from build123d import *

# Parameters (mm, degrees)
SKETCH2_W           = 20.32
SKETCH2_H           = 20.32
SKETCH2_R           = 1.325
BOSS_EXTRUDE1_DEPTH = 1.65
SKETCH3_W           = 0.55
SKETCH3_H           = 0.55
LPATTERN1_COUNT     = 4
LPATTERN1_PITCH     = 2.55
LPATTERN1_COL_COUNT = 4
LPATTERN1_COL_PITCH = 2.55
SKETCH5_W           = 17.9
SKETCH5_H           = 2.5
BOSS_EXTRUDE2_DEPTH = 2.75
SKETCH6_W           = 2
SKETCH6_H           = 2.5
SKETCH6_W_2         = 2.5
SKETCH6_H_2         = 3.5
BOSS_EXTRUDE3_DEPTH = 0.5
FILLET1_R           = 2
SKETCH7_W           = 1.7
SKETCH7_H           = 2.7
CUT_EXTRUDE1_DEPTH  = 0.1


with BuildPart() as part:
    # Sketch2 → Boss-Extrude1 (new body)
    with BuildSketch(Plane(origin=(0, 0, 0), x_dir=(1, 0, 0), z_dir=(0, 1, 0))):
        with Locations((10.16, 10.16)):
            Rectangle(SKETCH2_W, SKETCH2_H)
        with Locations((2.54, 17.695)):
            Circle(SKETCH2_R, mode=Mode.SUBTRACT)
        with Locations((17.78, 17.695)):
            Circle(SKETCH2_R, mode=Mode.SUBTRACT)
    extrude(amount=BOSS_EXTRUDE1_DEPTH)

    # Sweep1: sweep along a path in Sketch4
    with BuildLine(Plane(origin=(0, 0, 0), x_dir=(0, 0, -1), z_dir=(1, 0, 0))) as sweep1_path:
        Line((1.524, 1.65), (1.524, 5.25))
        ThreePointArc((1.524, 5.25), (1.231106781, 5.957106781), (0.524, 6.25))
        Line((0.524, 6.25), (-5.976, 6.25))
    # Sketch3 → Sweep1 (sweep)
    with BuildSketch(Plane(origin=(0, 1.65, 0), x_dir=(1, 0, 0), z_dir=(0, 1, 0))):
        with Locations((10.16, 1.524)):
            Rectangle(SKETCH3_W, SKETCH3_H)
    sweep1 = sweep(path=sweep1_path.line)

    # LPattern1: Sweep1 ×4
    with Locations(*[(-i * LPATTERN1_PITCH, 0, 0) for i in range(1, LPATTERN1_COUNT)]):
        add(sweep1)

    # LPattern1 col: Sweep1 ×4
    with Locations(*[(i * LPATTERN1_COL_PITCH, 0, 0) for i in range(1, LPATTERN1_COL_COUNT)]):
        add(sweep1)

    # Sketch5 → Boss-Extrude2 (add)
    with BuildSketch(Plane(origin=(0, 1.65, 0), x_dir=(1, 0, 0), z_dir=(0, 1, 0))):
        with Locations((10.16, 1.524)):
            Rectangle(SKETCH5_W, SKETCH5_H)
    extrude(amount=BOSS_EXTRUDE2_DEPTH)

    # Sketch6 → Boss-Extrude3 (add)
    with BuildSketch(Plane.XZ):
        with Locations((9.906, -9.906)):
            Rectangle(SKETCH6_W, SKETCH6_H)
        with Locations((13.208, -10.406)):
            Rectangle(SKETCH6_W_2, SKETCH6_H_2)
    extrude(amount=BOSS_EXTRUDE3_DEPTH)

    # Fillet1
    fillet1_edges = [part.edges().sort_by_distance(p)[0] for p in [
        (0, 0.825, -20.32),
        (20.32, 0.825, -20.32),
        (20.32, 0.825, 0),
        (0, 0.825, 0),
    ]]
    fillet(fillet1_edges, radius=FILLET1_R)

    # Sketch7 → Cut-Extrude1 (cut)
    with BuildSketch(Plane.XZ.offset(0.5)):
        with Locations((13.208, -10.406)):
            Rectangle(SKETCH7_W, SKETCH7_H)
    extrude(amount=-CUT_EXTRUDE1_DEPTH, mode=Mode.SUBTRACT)


solid = part.part
Read the model definition and answer for the solid it produces. Units are mm, in the model's axes. A direction names the side the tool comes from. Coordinates: 2 decimals unless noted, no trailing zeros. Loops run counter-clockwise (first coordinate to the right, second up) from the corner with the lowest first, then second, coordinate; pieces in that order, holes last. Notation, with made-up numbers: (15, 33.5) -> (58, 33.5) arc R20 ccw to (58, 55.5) -> close; hole circle Ø5 at (-25.75, 32.25). An arc over 180 degrees is marked (long way). Write item = value, one per line. Start each with the question number.
1) The part is cut by section C-C, the plane y = 6.25. Determine the outline of the cut face in (x, z) (3 decimals), plus the area to 3 significant figures.
2) Find the intervals of material crossed by L1, parallel to Z at x = 2.54, y = 0.7; L2, parallel to Y at x = 4.5, z = -12.25; L3, parallel to Z at x = 2.25, y = 3.25, in increasing order. Write a range as from..to.
3) The mould has two halves that part along X. Classify faces 6 (the face through (10, 1, 0)), 7 (the face through (19.72, 0.84, -19.75)), 8 (the face through (2.37, 0.81, -19.01)): pulls with the +X half, pulls with the -X half, needs draft (parallel to the pull), parting line crosses it, or undercut.
4) The part is cut by section A-A, the plane z = 3.75. Determine the outline of the cut face in (x, y) (3 decimals), plus the area to 3 significant figures.
5) The part is cut by section B-B, the plane x = 11.25. Determine the outline of the cut face in (y, z), plus the area to 3 significant figures.
6) For faces 1 (the face through (7.885, 6.2, 1.5)), 2 (the face through (10, 3, -0.274)), 3 (the face through (19.11, 3, -2)), 4 (the face through (13, -0.4, -10)), 5 (the face through (7.606, 6.142, -1.435)), determine the directions among +Z, -Z, +X, -X, +Y, -Y from which every point of the face is accessible in a straight line to the end or side of a thin tool.
7) Given P1, Ø2, axis at x = 13.5, y = 4.5, coming from the +Z side; P2, Ø1.1, axis at y = 5, z = 4, coming from the -X side; P3, Ø4, axis at x = 9.5, z = -15, coming from the -Y side; P4, Ø2.5, axis at y = 6, z = 2, coming from the -X side (3 decimals), each flat-ended and moving along its own axis, determine where each tip first touches the part or whether it passes through.
8) The part is cut by section D-D, the plane y = 0.5. Determine the outline of the cut face in (x, z) (3 decimals).
Result:
q1.outline = (2.235, -1.315) -> (2.785, -1.315) -> (2.785, 5.976) -> (2.235, 5.976) -> close; (4.785, -1.315) -> (5.335, -1.315) -> (5.335, 5.976) -> (4.785, 5.976) -> close; (7.335, -1.315) -> (7.885, -1.315) -> (7.885, 5.976) -> (7.335, 5.976) -> close; (9.885, -1.315) -> (10.435, -1.315) -> (10.435, 5.976) -> (9.885, 5.976) -> close; (12.435, -1.315) -> (12.985, -1.315) -> (12.985, 5.976) -> (12.435, 5.976) -> close; (14.985, -1.315) -> (15.535, -1.315) -> (15.535, 5.976) -> (14.985, 5.976) -> close; (17.535, -1.315) -> (18.085, -1.315) -> (18.085, 5.976) -> (17.535, 5.976) -> close
q1.area = 28.1 mm²
q2.L1 = -20.32..-19.02, -16.37..0
q2.L2 = 0..1.65
q2.L3 = -2.77..-0.27
q3.face_6 = needs draft
q3.face_7 = pulls with the +X half
q3.face_8 = undercut
q4.outline = (2.235, 5.975) -> (2.785, 5.975) -> (2.785, 6.525) -> (2.235, 6.525) -> close; (4.785, 5.975) -> (5.335, 5.975) -> (5.335, 6.525) -> (4.785, 6.525) -> close; (7.335, 5.975) -> (7.885, 5.975) -> (7.885, 6.525) -> (7.335, 6.525) -> close; (9.885, 5.975) -> (10.435, 5.975) -> (10.435, 6.525) -> (9.885, 6.525) -> close; (12.435, 5.975) -> (12.985, 5.975) -> (12.985, 6.525) -> (12.435, 6.525) -> close; (14.985, 5.975) -> (15.535, 5.975) -> (15.535, 6.525) -> (14.985, 6.525) -> close; (17.535, 5.975) -> (18.085, 5.975) -> (18.085, 6.525) -> (17.535, 6.525) -> close
q4.area = 2.12 mm²
q5.outline = (0, -20.32) -> (1.65, -20.32) -> (1.65, -2.77) -> (4.4, -2.77) -> (4.4, -0.27) -> (1.65, -0.27) -> (1.65, 0) -> (0, 0) -> close
q5.area = 40.4 mm²
q6.face_1 = +Z, -Z, +Y
q6.face_2 = +Z, +X, -X
q6.face_3 = +Z, -Z, +X, +Y
q6.face_4 = -Y
q6.face_5 = -Z, +X, -X, +Y
q7.P1 = -0.27
q7.P2 = through
q7.P3 = 0
q7.P4 = 2.235
q8.outline = (0, -18.32) arc R2 ccw to (2, -20.32) -> (18.32, -20.32) arc R2 ccw to (20.32, -18.32) -> (20.32, -2) arc R2 ccw to (18.32, 0) -> (2, 0) arc R2 ccw to (0, -2) -> close; hole circle Ø2.65 at (2.54, -17.695); hole circle Ø2.65 at (17.78, -17.695)
